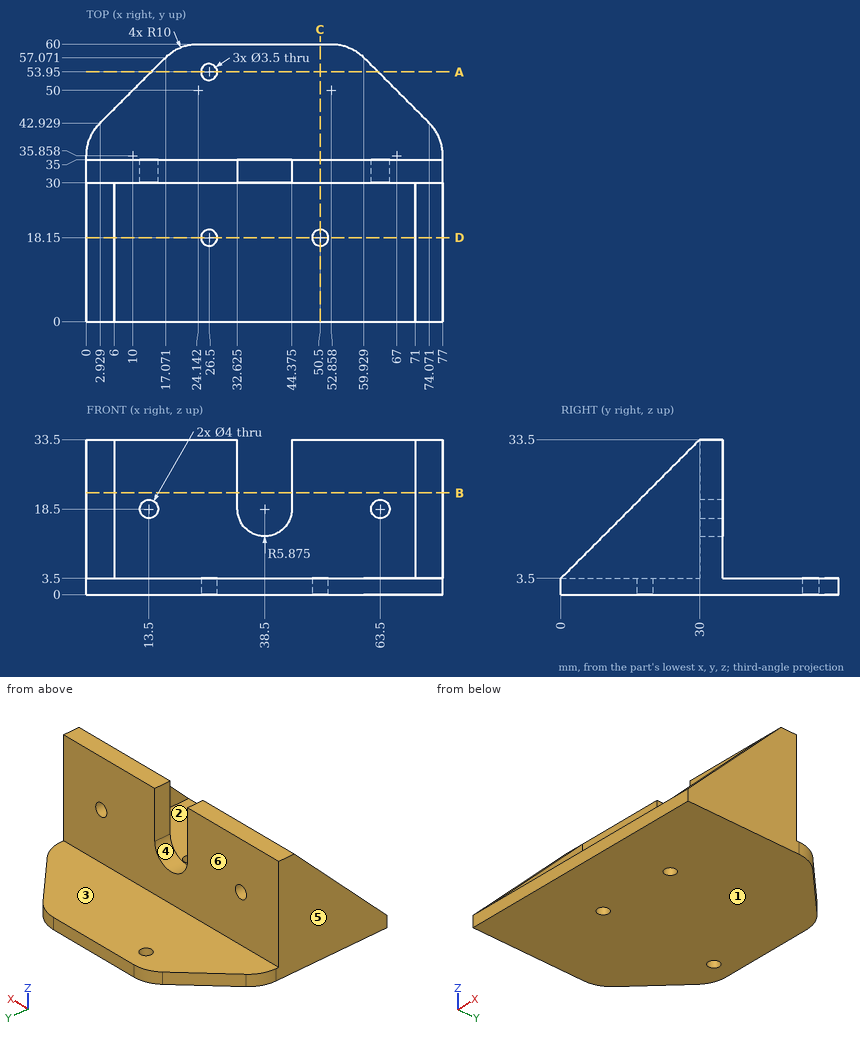
Verification items for this drawing (mm, ordinates from the low corner). A direction names the side the tool comes from. Coordinates: 2 decimals unless noted, no trailing zeros. Write each loop counter-clockwise with the first axis right and the second up, starting at its lowest first coordinate (ties: lowest second). Pieces come first, ordered by that corner, then holes. Notation, with made-up numbers: M -4.75,-19.5 L 8.25,-19.5 A24 ccw 8.25,-9.5 Z; hole C -22.5,-32.75 d8. An arc over 180 degrees is marked long. Answer as a JSON object with one key per item and string values. Group by question number.
(1) Material ranges on line 1 (X direction, y = 33.1, z = 18.5) (3 decimals); line 2 (Y direction, x = 50.5, z = 1.55); line 3 (Y direction, x = 26, z = 2), recorded low to high.
(2) Cross-section at D-D, the plane y = 18.15. Record the cut outline in (x, z), and give its area (3 significant figures).
(3) Cross-section at B-B, the plane z = 22. Record the cut outline in (x, y) (3 decimals).
(4) Gauge pin test, flat ends, axial feed: pin 1 (20 mm diameter, centred on x = 38, y = 49, fed in from +Z); pin 2 (3 mm diameter, centred on x = 43.5, z = 25, fed in from -Y); pin 3 (4 mm diameter, centred on x = 27, z = 8, fed in from +Y). Record the tip position at first contact, or that the pin passes through.
(5) Cross-section at A-A, the plane y = 53.95. Record the cut outline in (x, z).
(6) Tool access check on the marked faces 1, 2 and 3. Record the directions out of +Z, -Z, +X, -X, +Y, -Y that give a thin tool (end or side, any length) a straight path to the whole face; none if there is none.
(7) Release check for a two-part mould opening along X. For the marked faces 4, 5 and 6 record: +X half, -X half, draft (parallel to the pull), parting line (faces both ways), or undercut.
(8) Cross-section at C-C, the plane x = 50.5. Record the cut outline in (y, z).
Reply:
{
 "1": {"line 1": "0 to 11.5, 15.5 to 32.625, 44.375 to 61.5, 65.5 to 77", "line 2": "0 to 16.4, 19.9 to 60", "line 3": "0 to 16.47, 19.83 to 52.27, 55.63 to 60"},
 "2": {"outline": "M 0,0 L 24.75,0 L 24.75,3.5 L 6,3.5 L 6,21.65 L 0,21.65 Z; M 28.25,0 L 48.75,0 L 48.75,3.5 L 28.25,3.5 Z; M 52.25,0 L 77,0 L 77,21.65 L 71,21.65 L 71,3.5 L 52.25,3.5 Z", "area": "463 mm²"},
 "3": {"outline": "M 0,18.5 L 6,18.5 L 6,30 L 32.625,30 L 32.625,35 L 0,35 Z; M 44.375,30 L 71,30 L 71,18.5 L 77,18.5 L 77,35 L 44.375,35 Z"},
 "4": {"pin 1": "z = 3.5", "pin 2": "y = 30", "pin 3": "y = 35"},
 "5": {"outline": "M 13.95,0 L 24.75,0 L 24.75,3.5 L 13.95,3.5 Z; M 28.25,0 L 63.05,0 L 63.05,3.5 L 28.25,3.5 Z"},
 "6": {"face 1": "-Z, +X, -X, +Y, -Y", "face 2": "+Z, -Y", "face 3": "+Z, +X, -X, +Y"},
 "7": {"face 4": "undercut", "face 5": "-X half", "face 6": "draft"},
 "8": {"outline": "M 0,0 L 16.4,0 L 16.4,3.5 L 0,3.5 Z; M 19.9,0 L 60,0 L 60,3.5 L 35,3.5 L 35,33.5 L 30,33.5 L 30,3.5 L 19.9,3.5 Z"}
}
